```python
from build123d import *


with BuildPart() as part:
    # Sketch1 → Revolve1 (revolve)
    with BuildSketch(Plane.XY, mode=Mode.PRIVATE) as revolve1_sk:
        with BuildLine():
            Line((0, 7.09537037), (3.95, 7.09537037))
            ThreePointArc((3.95, 7.09537037), (3.576139111, 5.694289828), (2.438271605, 4.79537037))
            Line((2.438271605, 4.79537037), (3.557723263, -2.714506173))
            ThreePointArc((3.557723263, -2.714506173), (4.615478693, -4.037198455), (4.85, -5.714506173))
            Line((4.85, -5.714506173), (0.6, -5.714506173))
            Line((0.6, -5.714506173), (0.6, -14.714506173))
            Line((0.6, -14.714506173), (0, -16.561116295))
            Line((0, -16.561116295), (0, 7.09537037))
        make_face()
    revolve(revolve1_sk.sketch.rotate(Axis((0, 7.09537037, 0), (0, -1, 0)), 90), axis=Axis((0, 7.09537037, 0), (0, -1, 0)))


solid = part.part
```
Can you work these out from the model? Positions are in its coordinate system, mm. Coordinates: 2 decimals unless noted, no trailing zeros. Loops run counter-clockwise (first coordinate to the right, second up) from the corner with the lowest first, then second, coordinate; pieces in that order, holes last. Notation, with made-up numbers: M 8.5,-8 L 28.5,-8 A12 ccw 28.5,10 Z; hole C 53,33.5 d7. An arc over 180 degrees is marked long. Put each result on its own line as item: value. Start each with the question number.
(1) Imagine slicing it at A-A on y = -12.5. List the corners of the cut face in (x, z) for me, and give its area (3 significant figures).
(2) Will these pins go through, and if not, where does the flat tip stop? pin 1 Ø2 at (x, y) = (-0.5, 3) entering from +Z; pin 2 Ø5 at (x, z) = (-3.5, 1.5) entering from -Y.
(3) I need wall thicknesses on probe 1 along Y at (x, z) = (1, 0); probe 2 along X at (y, z) = (-3.75, -4); probe 3 along X at (y, z) = (-3, 3.5). Which ranges of each line are inside material? Lowest first, please.
(4) We'd pull the mould along Y, two halves only. Please class faces 1 (the face through (1.104, 1.822, 2.662)), 2 (the face through (0, -5.715, 1)), 3 (the face through (-0.506, -10.278, 0.323)), 4 (the face through (0, 7.095, 0)): +Y half, -Y half, draft (parallel to the pull), parting line (faces both ways), or undercut.
(5) Imagine slicing it at B-B on y = -2. List the corners of the cut face in (x, z) for me, and give its area (3 significant figures).
Worked answers:
1. outline: C 0,0 d1.2
1. area: 1.13 mm2
2. pin 1: stops at z = 2.84
2. pin 2: stops at y = -5.71
3. probe 1: y = -5.71 to 7.1
3. probe 2: x = -2 to 2
3. probe 3: x = -1.72 to 1.72
4. face 1: undercut
4. face 2: -Y half
4. face 3: draft
4. face 4: +Y half
5. outline: C 0,0 d6.9
5. area: 37.4 mm2
